Work out the finished part from the listing and answer in its coordinate system (mm). Coordinates: 2 decimals unless noted, no trailing zeros. Order: outer loops, then holes, each group sorted by start corner. A loop starts at its lowest first (then second) coordinate and runs counter-clockwise, first axis right, second up. Notation, with made-up numbers: M 16,0.25 L 32,0.25 A11 cw 32,20.25 Z; hole C 8.25,-24.75 d5. An arc over 180 degrees is marked long. Use a Markdown table: item, result. Add a question column.
Autodesk Inventor part; units mm, degrees
ref_plane "YZ Plane" through (0, 0, 0) normal (1, 0, 0) x (0, 1, 0)
ref_plane "XZ Plane" through (0, 0, 0) normal (0, 1, 0) x (-1, 0, 0)
ref_plane "XY Plane" through (0, 0, 0) normal (0, 0, 1) x (1, 0, 0)
ref_plane "РабПлоскость1" through (0, 0, 0) normal (0, 0, 1) x (1, 0, 0)
sketch "Эскиз1" plane through (0, 0, 0) normal (0, 0, 1) x (1, 0, 0)
  line L0 (-134.636, 128) -> (-134.636, -128)
  arc A0 (-134.636, -128) -> (-132.636, -130) centre (-132.636, -128) ccw
  line L1 (-132.636, -130) -> (132.636, -130)
  arc A1 (132.636, -130) -> (134.636, -128) centre (132.636, -128) ccw
  line L2 (134.636, -128) -> (134.636, 128)
  arc A2 (134.636, 128) -> (132.636, 130) centre (132.636, 128) ccw
  line L3 (132.636, 130) -> (-132.636, 130)
  arc A3 (-132.636, 130) -> (-134.636, 128) centre (-132.636, 128) ccw
  circle A4 centre (-124.636, 120) radius 4
  circle A5 centre (-0.636, 120) radius 4
  circle A6 centre (123.364, 120) radius 4
  circle A7 centre (123.364, 60) radius 4
  circle A8 centre (123.364, 0) radius 4
  circle A9 centre (-124.636, -60) radius 4
  circle A10 centre (123.364, -60) radius 4
  circle A11 centre (-124.636, -120) radius 4
  circle A12 centre (-62.636, -120) radius 4
  circle A13 centre (-0.636, -120) radius 4
  circle A14 centre (61.364, -120) radius 4
  circle A15 centre (123.364, -120) radius 4
  circle A16 centre (-124.636, 0) radius 4
  circle A17 centre (-124.636, 60) radius 4
  circle A18 centre (61.364, 120) radius 4
  circle A19 centre (-62.636, 120) radius 4
  line L4 (115.364, 110) -> (115.364, -110)
  line L5 (115.364, -110) -> (-114.636, -110)
  line L6 (-114.636, -110) -> (-114.636, 110)
  line L7 (-114.636, 110) -> (115.364, 110)
  point P0 (0, 0)
extrude "Выдавливание1" add sketch "Эскиз1" along normal blind 5 contours A3 L3 A2 L2 A1 L1 A0 L0 | L4 L5 L6 L7
properties part number "Крышка водяной рубашки" material "Чугун, серый"
(1) A cutting plane is placed at B-B on y = 0. Write down the section's boundary in (x, z).
(2) The mould has two halves that part along Y. Classify faces 1 (the flat face through (-2, 2, 0)), 2 (the cylindrical face through (-1.157, -123.966, 2.465)): pulls with the +Y half, pulls with the -Y half, needs draft (parallel to the pull), parting line crosses it, or undercut.
(3) A cutting plane is placed at A-A on y = -120. Write down the section's boundary in (x, z), plus the area to 3 significant figures.
(4) Straight lines are drawn through the part: line 1 (Y direction, x = -63.5, z = 0.65); line 2 (Y direction, x = -61.5, z = 2.55); line 3 (X direction, y = -59, z = 2.55). For each, find the intervals that lie inside material, in ascending order.
(5) Given P1, Ø7, axis at x = 123.364, y = -120, coming from the +Z side, flat-ended and moving along its own axis, determine where the tip first touches the part or whether it passes through.
From the geometry:
| question | item | result |
|---|---|---|
| 1 | outline | M -134.64,0 L -128.64,0 L -128.64,5 L -134.64,5 Z; M -120.64,0 L 119.36,0 L 119.36,5 L -120.64,5 Z; M 127.36,0 L 134.64,0 L 134.64,5 L 127.36,5 Z |
| 2 | face 1 | needs draft |
| 2 | face 2 | undercut |
| 3 | outline | M -134.64,0 L -128.64,0 L -128.64,5 L -134.64,5 Z; M -120.64,0 L -66.64,0 L -66.64,5 L -120.64,5 Z; M -58.64,0 L -4.64,0 L -4.64,5 L -58.64,5 Z; M 3.36,0 L 57.36,0 L 57.36,5 L 3.36,5 Z; M 65.36,0 L 119.36,0 L 119.36,5 L 65.36,5 Z; M 127.36,0 L 134.64,0 L 134.64,5 L 127.36,5 Z |
| 3 | area | 1,150 mm2 |
| 4 | line 1 | y = -130 to -123.91, -116.09 to 116.09, 123.91 to 130 |
| 4 | line 2 | y = -130 to -123.84, -116.16 to 116.16, 123.84 to 130 |
| 4 | line 3 | x = -134.64 to -128.51, -120.76 to 119.49, 127.24 to 134.64 |
| 5 | P1 | passes through |
